Design review of the part shown in the three views and the two pictorial views. Dimensions are in mm from the part's minimum x, y and z. Coordinates: 2 decimals unless noted, no trailing zeros. Loops run counter-clockwise (first coordinate to the right, second up) from the corner with the lowest first, then second, coordinate; pieces in that order, holes last. Notation, with made-up numbers: (-13.5, 65) - (45.5, 65) arc R15 ccw to (45.5, 74) - close; hole circle Ø1 at (4.25, 38.25). An arc over 180 degrees is marked (long way). One line per question, with ' | ' between items.
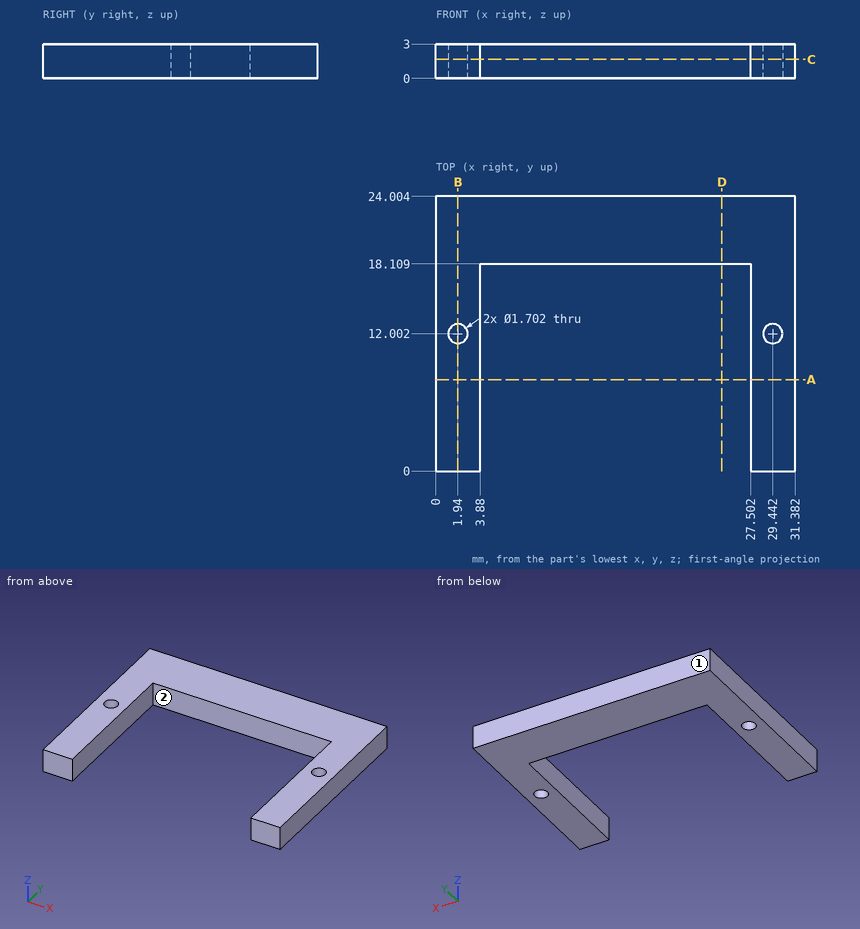
Q1. Draft analysis for pull direction X (two halves, no side actions). For the marked faces 1 and 2, state which applies: +X half, -X half, draft (parallel to the pull), parting line (faces both ways), or undercut.
Returned:
face 1: draft | face 2: undercut
Q2. Take a section at B-B (x = 1.94). Give the boundary of the cut face in (y, z), plus the area to 3 significant figures.
Returned:
outline: (0, 0) - (11.15, 0) - (11.15, 3) - (0, 3) - close; (12.85, 0) - (24, 0) - (24, 3) - (12.85, 3) - close | area: 66.9 mm²
Q3. Take a section at C-C (z = 1.65). Give the boundary of the cut face in (x, y), plus the area to 3 significant figures.
Returned:
outline: (0, 0) - (3.88, 0) - (3.88, 18.11) - (27.5, 18.11) - (27.5, 0) - (31.38, 0) - (31.38, 24) - (0, 24) - close; hole circle Ø1.7 at (1.94, 12); hole circle Ø1.7 at (29.44, 12) | area: 321 mm²
Q4. Take a section at A-A (y = 8). Give the boundary of the cut face in (x, z), plus the area to 3 significant figures.
Returned:
outline: (0, 0) - (3.88, 0) - (3.88, 3) - (0, 3) - close; (27.5, 0) - (31.38, 0) - (31.38, 3) - (27.5, 3) - close | area: 23.3 mm²
Q5. For pin 1 (1.5 mm diameter, centred on y = 6, z = 2.5, fed in from -X); pin 2 (1 mm diameter, centred on x = 8.5, z = 1.5, fed in from -Y), all flat-tipped, find the tip position at first contact; note any pin that passes through.
Returned:
pin 1: stops at x = 0 | pin 2: stops at y = 18.11
Q6. To check wall thickness, follow line 1 along X through (y, z) = (3.5, 0.55); line 2 along Y through (x, z) = (1.94, 0.95); line 3 along X through (y, z) = (11.5, 0.8) (1 decimal). State the ranges of each line that lie inside material, in increasing order.
Returned:
line 1: x = 0 to 3.88, 27.5 to 31.38 | line 2: y = 0 to 11.15, 12.85 to 24 | line 3: x = 0 to 1.3, 2.6 to 3.9, 27.5 to 28.8, 30.1 to 31.4
Q7. Take a section at D-D (x = 25). Give the boundary of the cut face in (y, z), plus the area to 3 significant figures.
Returned:
outline: (18.11, 0) - (24, 0) - (24, 3) - (18.11, 3) - close | area: 17.7 mm²
